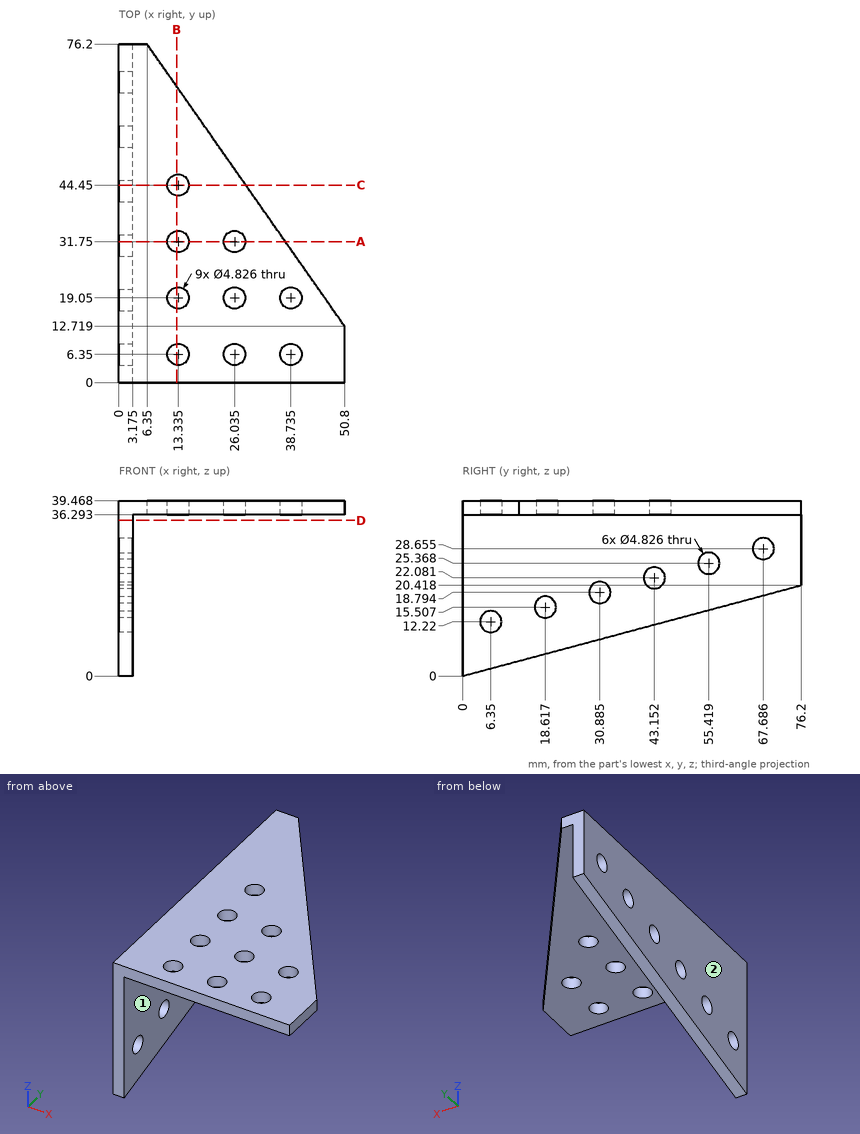
Here's the drawing with two shaded views (mm, measured from the low corner). I have some questions. A direction names the side the tool comes from. Coordinates: 2 decimals unless noted, no trailing zeros. Loops run counter-clockwise (first coordinate to the right, second up) from the corner with the lowest first, then second, coordinate; pieces in that order, holes last. Notation, with made-up numbers: M -17,48 L -12,48 A10 cw -12,52 Z; hole C -8.75,-3.75 d4. An arc over 180 degrees is marked long. Return JSON: item names as keys, results as strings. Group by question number.
Item 1: On a 3-axis mill with a long thin cutter (end or side, diameter ignored), from which of +Z, -Z, +X, -X, +Y, -Y can I reach the whole of each face in a straight line? I mean the marked faces 1 and 2. Say none if no direction works.
Item 2: Imagine slicing it at D-D (z = 35). Please give me the cut outline in (x, y) (1 decimal), and give its area (3 significant figures).
Item 3: If I drill on L1, parallel to X at y = 26.5, z = 26.5 (1 decimal); L2, parallel to X at y = 44, z = 38 (1 decimal); L3, parallel to Z at x = 12, y = 14.5, over which ranges is the centre line in solid material (lowest first)? Write a range as from..to.
Item 4: Imagine slicing it at C-C (y = 44.45). Please give me the cut outline in (x, z) (1 decimal), and give its area (3 significant figures).
Item 5: Imagine slicing it at A-A (y = 31.75). Please give me the cut outline in (x, z) (1 decimal).
Item 6: I'm going to push flat-ended pins straight in: pin 1 Ø5.5 at (x, y) = (13.335, 19.05) entering from -Z; pin 2 Ø1.5 at (y, z) = (9.5, 5.5) entering from +X (1 decimal). Where does each tip first touch, or does it pass through?
Item 7: Imagine slicing it at B-B (x = 13). Please give me the cut outline in (y, z), and give its area (3 significant figures).
Verdict:
{
 "1": {"face 1": "-Z, +X, +Y, -Y", "face 2": "+Z, -Z, -X, +Y, -Y"},
 "2": {"outline": "M 0,0 L 3.2,0 L 3.2,76.2 L 0,76.2 Z", "area": "242 mm^2"},
 "3": {"L1": "x = 0..3.2", "L2": "x = 0..11, 15.7..28.9", "L3": "z = 36.29..39.47"},
 "4": {"outline": "M 0,11.9 L 3.2,11.9 L 3.2,20 L 0,20 Z; M 0,24.1 L 3.2,24.1 L 3.2,36.3 L 10.9,36.3 L 10.9,39.5 L 0,39.5 Z; M 15.7,36.3 L 28.6,36.3 L 28.6,39.5 L 15.7,39.5 Z", "area": "140 mm^2"},
 "5": {"outline": "M 0,8.5 L 3.2,8.5 L 3.2,16.5 L 0,16.5 Z; M 0,21 L 3.2,21 L 3.2,36.3 L 10.9,36.3 L 10.9,39.5 L 0,39.5 Z; M 15.7,36.3 L 23.6,36.3 L 23.6,39.5 L 15.7,39.5 Z; M 28.4,36.3 L 37.5,36.3 L 37.5,39.5 L 28.4,39.5 Z"},
 "6": {"pin 1": "stops at z = 36.29", "pin 2": "stops at x = 3.2"},
 "7": {"outline": "M 0,36.29 L 3.96,36.29 L 3.96,39.47 L 0,39.47 Z; M 8.74,36.29 L 16.66,36.29 L 16.66,39.47 L 8.74,39.47 Z; M 21.44,36.29 L 29.36,36.29 L 29.36,39.47 L 21.44,39.47 Z; M 34.14,36.29 L 42.06,36.29 L 42.06,39.47 L 34.14,39.47 Z; M 46.84,36.29 L 66.7,36.29 L 66.7,39.47 L 46.84,39.47 Z", "area": "151 mm^2"}
}
